Autodesk Inventor part; units mm, degrees
ref_plane "YZ Plane" through (0, 0, 0) normal (1, 0, 0) x (0, 1, 0)
ref_plane "XZ Plane" through (0, 0, 0) normal (0, 1, 0) x (-1, 0, 0)
ref_plane "XY Plane" through (0, 0, 0) normal (0, 0, 1) x (1, 0, 0)
sketch "Sketch1" plane through (0, 0, 0) normal (0, 1, 0) x (-1, 0, 0)
  line L0 (12.5, 12.5) -> (12.5, -12.5)
  line L1 (12.5, -12.5) -> (-12.5, -12.5)
  line L2 (12.5, 12.5) -> (-12.5, 12.5)
  line L3 (-12.5, 12.5) -> (-12.5, -12.5)
  arc A0 (-2.489, -1.6837) -> (-2.489, 1.6837) centre (0, 0) ccw
  line L4 (-2.489, -1.6837) -> (-2.489, 1.6837)
  dimension "d8" = 12.5
  dimension "d9" = 25
  dimension "d10" = 12.5
  dimension "d11" = 25
  dimension "d12" = 6.01
  dimension "d13" = 2.489
extrude "Extrusion1" add sketch "Sketch1" along normal blind 20
sketch "Sketch2" plane through (-12.5, 0, 12.5) normal (0, 0, 1) x (1, 0, 0)
  circle A0 centre (5.2959, 14.7041) radius 4.6609 construction
  circle A1 centre (5.2959, 5.2959) radius 4.6609 construction
  circle A2 centre (19.7041, 14.7041) radius 4.6609 construction
  circle A3 centre (19.7041, 5.2959) radius 4.6609 construction
  line L0 (0, 0) -> (0, 20)
  line L1 (25, 0) -> (25, 20)
  line L2 (0, 20) -> (25, 20)
  line L3 (0, 0) -> (25, 0)
  line L4 (5.2959, 14.7041) -> (19.7041, 14.7041) construction
  line L5 (5.2959, 5.2959) -> (19.7041, 5.2959) construction
  line L6 (24.365, 14.7041) -> (22.0345, 10.6676)
  line L7 (22.0345, 10.6676) -> (17.3737, 10.6676)
  line L8 (17.3737, 10.6676) -> (15.0432, 14.7041)
  line L9 (15.0432, 14.7041) -> (17.3737, 18.7406)
  line L10 (17.3737, 18.7406) -> (22.0345, 18.7406)
  line L11 (22.0345, 18.7406) -> (24.365, 14.7041)
  line L12 (24.365, 5.2959) -> (22.0345, 1.2594)
  line L13 (22.0345, 1.2594) -> (17.3737, 1.2594)
  line L14 (17.3737, 1.2594) -> (15.0432, 5.2959)
  line L15 (15.0432, 5.2959) -> (17.3737, 9.3324)
  line L16 (17.3737, 9.3324) -> (22.0345, 9.3324)
  line L17 (22.0345, 9.3324) -> (24.365, 5.2959)
  line L18 (9.9568, 5.2959) -> (7.6264, 1.2594)
  line L19 (7.6264, 1.2594) -> (2.9655, 1.2594)
  line L20 (2.9655, 1.2594) -> (0.635, 5.2959)
  line L21 (0.635, 5.2959) -> (2.9654, 9.3324)
  line L22 (2.9654, 9.3324) -> (7.6263, 9.3324)
  line L23 (7.6263, 9.3324) -> (9.9568, 5.2959)
  line L24 (9.9568, 14.7041) -> (7.6264, 10.6676)
  line L25 (7.6264, 10.6676) -> (2.9655, 10.6676)
  line L26 (2.9655, 10.6676) -> (0.635, 14.7041)
  line L27 (0.635, 14.7041) -> (2.9654, 18.7406)
  line L28 (2.9654, 18.7406) -> (7.6263, 18.7406)
  line L29 (7.6263, 18.7406) -> (9.9568, 14.7041)
  point P0 (12.5, 0)
  dimension "d16" = 9.3218
  dimension "d17" = 9.3218
  dimension "d18" = 9.3218
  dimension "d19" = 9.3218
  dimension "d20" = 5.2959
  dimension "d21" = 5.2959
  dimension "d22" = 5.2959
  dimension "d23" = 5.2959
  dimension "d24" = 5.2959
  dimension "d25" = 5.2959
  dimension "d26" = 5.2959
  dimension "d27" = 5.2959
sketch "Sketch3" plane through (12.5, 0, -12.5) normal (0, 0, -1) x (-1, 0, 0)
  circle A0 centre (5.2959, 14.7041) radius 1.9304
  line L0 (0, 20) -> (25, 20)
  line L1 (0, 0) -> (0, 20)
  circle A1 centre (5.2959, 5.2959) radius 1.9304
  line L2 (0, 0) -> (25, 0)
  circle A2 centre (19.7041, 14.7041) radius 1.9304
  line L3 (25, 0) -> (25, 20)
  circle A3 centre (19.7041, 5.2959) radius 1.9304
  point P0 (12.5, 0)
  dimension "d28" = 3.8608
  dimension "d29" = 5.2959
  dimension "d30" = 5.2959
  dimension "d31" = 3.8608
  dimension "d32" = 5.2959
  dimension "d33" = 5.2959
  dimension "d34" = 3.8608
  dimension "d35" = 5.2959
  dimension "d36" = 5.2959
  dimension "d37" = 3.8608
  dimension "d38" = 5.2959
  dimension "d39" = 5.2959
extrude "6-32Holes" cut sketch "Sketch3" against normal through all contours A0 | A1 | A2 | A3
extrude "NutWells" cut sketch "Sketch2" against normal blind 4.3688 contours L6 L7 L8 L9 L10 L11 | L12 L13 L14 L15 L16 L17 | L18 L19 L20 L21 L22 L23 | L24 L25 L26 L27 L28 L29
equation "\"d20\" = d21"
equation "\"d22\" = d23"
equation "\"d24\" = d23"
equation "\"d25\" = d23"
equation "\"d26\" = d21"
equation "\"d27\" = d21"
equation "\"d29\" = d23"
equation "\"d30\" = d21"
equation "\"d31\" = d28"
equation "\"d32\" = d23"
equation "\"d33\" = d21"
equation "\"d34\" = d28"
equation "\"d35\" = d21"
equation "\"d36\" = d23"
equation "\"d37\" = d28"
equation "\"d38\" = d23"
equation "\"d39\" = d21"
properties part number "615456 bevel gear lock A"
Could you check a few things on this model? Use its own coordinates, in mm. A direction names the side the tool comes from. Give positions to 0.01 mm unless a question says otherwise; leave off trailing zeros. Order: outer loops, then holes, each group sorted by start corner. A loop starts at its lowest first (then second) coordinate and runs counter-clockwise, first axis right, second up. Notation, with made-up numbers: (50.5, -10.5) - (92.5, -10.5) arc R23 cw to (92.5, 21.5) - close; hole circle Ø2 at (-17, 7). An arc over 180 degrees is marked (long way). One line per item, written item: value. Start each with the question number.
1. Imagine slicing it at B-B on x = 0. List the corners of the cut face in (y, z) for me (3 decimals), plus the area to 3 significant figures.
2. Thinking about a two-plate mould opening in X: for faces 1 (the face through (12.5, 10, 0)), 2 (the face through (-3.7, 12.7, 10.3)), 3 (the face through (7, 9.332, 10)), 4 (the face through (-12.5, 10, 0)), which applies, +X half, -X half, draft (parallel to the pull), parting line (faces both ways), or undercut?
3. For faces 5 (the face through (3.69, 16.69, 10.35)), 6 (the face through (-6.79, 12.82, -2.33)), which set-ups out of +Z, -Z, +X, -X, +Y, -Y let a thin tool reach every point of the face, with its end or its side?
4. Imagine slicing it at A-A on z = 0. List the corners of the cut face in (x, y) for me (1 decimal), plus the area to 3 significant figures.
5. If I drill on probe 1 along X at (y, z) = (14.75, -4.25); probe 2 along X at (y, z) = (8.25, 11); probe 3 along Y at (x, z) = (7.5, -6.75), over which ranges is the centre line in solid material (lowest first)?
6. Imagine slicing it at D-D on z = -4.25. List the corners of the cut face in (x, y) for me.
7. Imagine slicing it at C-C on y = 6. List the corners of the cut face in (x, z) for me.
8. For P1, Ø2.5, axis at x = 7.2, y = 14.7, coming from the +Z side, with a flat end and sliding along its axis, tell me the tip position at first contact or that it passes through.
Values:
1. outline: (0, -12.5) - (20, -12.5) - (20, -3.005) - (0, -3.005) - close; (0, 3.005) - (20, 3.005) - (20, 12.5) - (0, 12.5) - close
1. area: 380 mm²
2. face 1: +X half
2. face 2: undercut
2. face 3: undercut
2. face 4: -X half
3. face 5: +Z
3. face 6: +Z, -Z
4. outline: (-12.5, 0) - (-3, 0) - (-3, 20) - (-12.5, 20) - close; (2.5, 0) - (12.5, 0) - (12.5, 20) - (2.5, 20) - close; hole circle Ø3.9 at (-7.2, 5.3); hole circle Ø3.9 at (-7.2, 14.7); hole circle Ø3.9 at (7.2, 5.3); hole circle Ø3.9 at (7.2, 14.7)
4. area: 343 mm²
5. probe 1: -12.5 to -9.13, -5.27 to 5.27, 9.13 to 12.5
5. probe 2: -12.5 to -10.16, -4.25 to 4.25, 10.16 to 12.5
5. probe 3: 0 to 3.39, 7.2 to 12.8, 16.61 to 20
6. outline: (-12.5, 0) - (12.5, 0) - (12.5, 20) - (-12.5, 20) - close; hole circle Ø3.86 at (-7.2, 5.3); hole circle Ø3.86 at (-7.2, 14.7); hole circle Ø3.86 at (7.2, 5.3); hole circle Ø3.86 at (7.2, 14.7)
7. outline: (-12.5, -12.5) - (-9, -12.5) - (-9, 8.13) - (-11.46, 8.13) - (-11.46, 12.5) - (-12.5, 12.5) - close; (-5.41, -12.5) - (5.41, -12.5) - (5.41, 8.13) - (2.95, 8.13) - (2.95, 12.5) - (-2.95, 12.5) - (-2.95, 8.13) - (-5.41, 8.13) - close; (9, -12.5) - (12.5, -12.5) - (12.5, 12.5) - (11.46, 12.5) - (11.46, 8.13) - (9, 8.13) - close; hole (2.49, -1.68) - (2.49, 1.68) arc R3 ccw (long way) to start
8. P1: through
